For this review, take the finished solid that the model builds, in its own axes (mm). Face numbers are marked on the shaded views. A direction names the side the tool comes from. Round coordinates to 2 decimals unless told otherwise and drop trailing zeros. Order: outer loops, then holes, each group sorted by start corner. A loop starts at its lowest first (then second) coordinate and runs counter-clockwise, first axis right, second up. Notation, with made-up numbers: (32, -4) - (71, -4) arc R14 cw to (71, 12) - close; hole circle Ø3 at (54, 20). An arc over 180 degrees is marked (long way). One line per item, written item: value.
```python
from build123d import *

# Parameters (mm, degrees)
SKETCH1_R           = 10.25
BOSS_EXTRUDE1_DEPTH = 12
SKETCH2_R           = 3
CUT_EXTRUDE1_DEPTH  = 8
SKETCH3_R           = 15
CUT_EXTRUDE2_DEPTH  = 5
BOSS_EXTRUDE2_DEPTH = 12
FILLET2_R           = 5


with BuildPart() as part:
    # Sketch1 → Boss-Extrude1 (new body)
    with BuildSketch(Plane.XY):
        with BuildLine():
            Line((-10.535653753, -17), (-37, -17))
            Line((-37, -17), (-37, -24))
            Line((-37, -24), (0, -24))
            Line((0, -24), (37, -24))
            Line((37, -24), (37, -17))
            Line((37, -17), (10.535653753, -17))
            ThreePointArc((10.535653753, -17), (0, 20), (-10.535653753, -17))
        make_face()
        Circle(SKETCH1_R, mode=Mode.SUBTRACT)
    extrude(amount=BOSS_EXTRUDE1_DEPTH)

    # Sketch2 → Cut-Extrude1 (cut, through all)
    with BuildSketch(Plane(origin=(0, -17, 0), x_dir=(1, 0, 0), z_dir=(0, 1, 0))):
        with Locations((30, -6)):
            Circle(SKETCH2_R)
        with Locations((-30, -6)):
            Circle(SKETCH2_R)
    extrude(amount=-CUT_EXTRUDE1_DEPTH, mode=Mode.SUBTRACT)

    # Sketch3 → Cut-Extrude2 (cut)
    with BuildSketch(Plane(origin=(0, 0, 0), x_dir=(-1, 0, 0), z_dir=(0, 0, -1))):
        Circle(SKETCH3_R)
    extrude(amount=-CUT_EXTRUDE2_DEPTH, mode=Mode.SUBTRACT)

    # Sketch4 → Boss-Extrude2 (add, through all)
    with BuildSketch(Plane(origin=(0, 0, 0), x_dir=(-1, 0, 0), z_dir=(0, 0, -1))):
        Polygon((-20, 0), (-10.535653753, -17), (-20, -17), align=None)
        Polygon((20, 0), (20, -17), (10.535653753, -17), align=None)
    extrude(amount=-BOSS_EXTRUDE2_DEPTH)

    # Fillet2
    fillet2_edges = [part.edges().sort_by_distance(p)[0] for p in [
        (-20, -17, 6),
        (20, -17, 6),
    ]]
    fillet(fillet2_edges, radius=FILLET2_R)


solid = part.part
```
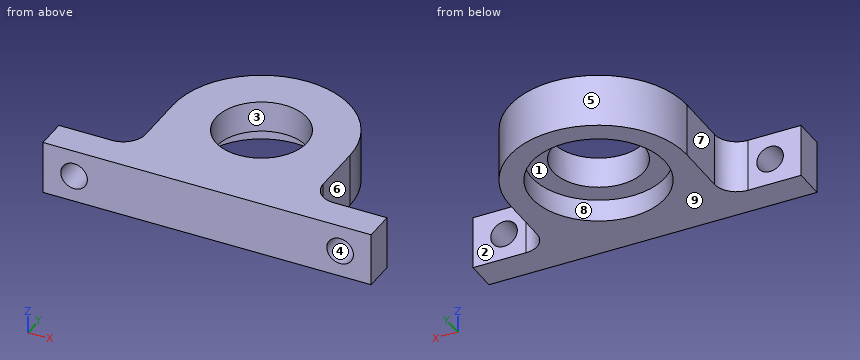
Item 1: Take a section at D-D (y = 2). Write out the cut boundary in (x, z), plus the area to 3 significant figures.
Returned:
outline: (-19.9, 0) - (-14.87, 0) - (-14.87, 5) - (-10.05, 5) - (-10.05, 12) - (-19.9, 12) - close; (10.05, 5) - (14.87, 5) - (14.87, 0) - (19.9, 0) - (19.9, 12) - (10.05, 12) - close
area: 188 mm^2
Item 2: Take a section at C-C (z = 10). Write out the cut boundary in (x, y).
Returned:
outline: (-37, -24) - (37, -24) - (37, -17) - (25, -17) arc R5 cw to (20, -12) - (20, 0) arc R20 ccw to (-20, 0) - (-20, -12) arc R5 cw to (-25, -17) - (-37, -17) - close; hole circle Ø20.5 at (0, 0)
Item 3: Take a section at A-A (z = 6). Write out the cut boundary in (x, y).
Returned:
outline: (-37, -24) - (-33, -24) - (-33, -17) - (-37, -17) - close; (-27, -24) - (27, -24) - (27, -17) - (25, -17) arc R5 cw to (20, -12) - (20, 0) arc R20 ccw to (-20, 0) - (-20, -12) arc R5 cw to (-25, -17) - (-27, -17) - close; (33, -24) - (37, -24) - (37, -17) - (33, -17) - close; hole circle Ø20.5 at (0, 0)
Item 4: For P1, Ø6, axis at x = -10.5, z = 6.5, coming from the +Y side; P2, Ø12, axis at x = -4.5, y = -3.5, coming from the -Z side; P3, Ø6, axis at x = 29.5, z = 3, coming from the +Y side, all flat-tipped, find the tip position at first contact; note any pin that passes through.
Returned:
P1: y = 18.54
P2: z = 5
P3: y = -17
Item 5: Wall thickness on line 1 (X direction, y = -19.75, z = 6); line 2 (Z direction, x = 30, y = -21); line 3 (X direction, y = 0, z = 10): over which ranges is each line inside the solid? List them lowest first.
Returned:
line 1: -37 to -33, -27 to 27, 33 to 37
line 2: 0 to 3, 9 to 12
line 3: -20 to -10.25, 10.25 to 20
Item 6: Machinability: for the marked faces 5, 6, 7, 8 and 9, which of the approach directions +Z, -Z, +X, -X, +Y, -Y give a long, thin tool a straight path to every point of the face, cutting with its end or side? Answer none if there is none.
Returned:
face 5: +Z, -Z, +Y
face 6: +Z, -Z, +X, +Y
face 7: +Z, -Z, -X, +Y
face 8: -Z
face 9: -Z, +X, -X, +Y, -Y
Item 7: Take a section at B-B (x = 0). Write out the cut boundary in (y, z).
Returned:
outline: (-24, 0) - (-15, 0) - (-15, 5) - (-10.25, 5) - (-10.25, 12) - (-24, 12) - close; (10.25, 5) - (15, 5) - (15, 0) - (20, 0) - (20, 12) - (10.25, 12) - close
Item 8: The part is to be moulded in two halves that separate along Y. For the marked faces 1, 2, 3 and 4, say which applies: +Y half, -Y half, draft (parallel to the pull), parting line (faces both ways), or undercut.
Returned:
face 1: undercut
face 2: +Y half
face 3: undercut
face 4: draft
